Part model, mm, in its own coordinate system. Face numbers are marked on the shaded views. A direction names the side the tool comes from. Round coordinates to 2 decimals unless told otherwise and drop trailing zeros. Loops run counter-clockwise (first coordinate to the right, second up) from the corner with the lowest first, then second, coordinate; pieces in that order, holes last. Notation, with made-up numbers: (-21.75, 80) - (-2.75, 80) arc R18 ccw to (-2.75, 101) - close; hole circle Ø1 at (-33.75, 80.5). An arc over 180 degrees is marked (long way). Put each result on its own line as item: value.
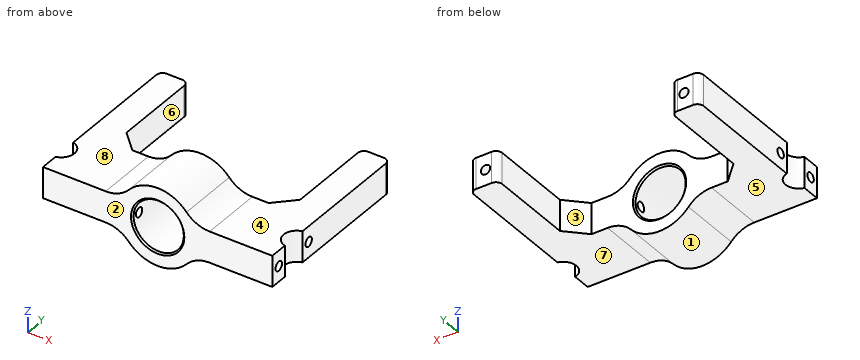
from build123d import *

# Parameters (mm, degrees)
SKETCH1_W                = 88
SKETCH1_H                = 10
BOSS_EXTRUDE1_DEPTH      = 20
SKETCH2_R                = 4.25
CUT_EXTRUDE1_DEPTH       = 11
SKETCH7_R                = 12.5
BOSS_EXTRUDE2_DEPTH      = 20
SKETCH4_R                = 8.1
CUT_EXTRUDE3_DEPTH       = 21
FILLET2_R                = 10
SKETCH9_W                = 7
SKETCH9_H                = 20
CUT_EXTRUDE6_DEPTH       = 18.5
SKETCH10_W               = 9
SKETCH10_H               = 10
BOSS_EXTRUDE3_DEPTH      = 35
SKETCH11_R               = 1.5
CUT_EXTRUDE7_DEPTH       = 20
CHAMFER1_SIZE            = 6
FILLET3_R                = 2
CHAMFER1_OF_MIRROR1_SIZE = 6
FILLET3_OF_MIRROR1_R     = 2
CHAMFER2_SIZE            = 0.5
SKETCH12_R               = 1.5
CUT_EXTRUDE8_DEPTH       = 75


with BuildPart() as part:
    # Sketch1 → Boss-Extrude1 (new body)
    with BuildSketch(Plane(origin=(0, 0, 0), x_dir=(1, 0, 0), z_dir=(0, 1, 0))):
        Rectangle(SKETCH1_W, SKETCH1_H)
    extrude(amount=BOSS_EXTRUDE1_DEPTH)

    # Sketch2 → Cut-Extrude1 (cut, through all)
    with BuildSketch(Plane.XY.offset(5)):
        with Locations((-38, 10)):
            Circle(SKETCH2_R)
        with Locations((38, 10)):
            Circle(SKETCH2_R)
    extrude(amount=-CUT_EXTRUDE1_DEPTH, mode=Mode.SUBTRACT)

    # Sketch7 → Boss-Extrude2 (add)
    with BuildSketch(Plane(origin=(0, 20, 0), x_dir=(1, 0, 0), z_dir=(0, 1, 0))):
        Circle(SKETCH7_R)
    extrude(amount=-BOSS_EXTRUDE2_DEPTH)

    # Sketch4 → Cut-Extrude3 (cut, through all)
    with BuildSketch(Plane(origin=(0, 20, 0), x_dir=(1, 0, 0), z_dir=(0, 1, 0))):
        Circle(SKETCH4_R)
    extrude(amount=-CUT_EXTRUDE3_DEPTH, mode=Mode.SUBTRACT)

    # Fillet2
    fillet2_edges = [part.edges().sort_by_distance(p)[0] for p in [
        (11.456439237, 10, -5),
        (11.456439237, 10, 5),
        (-11.456439237, 10, -5),
        (-11.456439237, 10, 5),
    ]]
    fillet(fillet2_edges, radius=FILLET2_R)

    # Sketch9 → Cut-Extrude6 (cut, through all)
    with BuildSketch(Plane.XY.offset(5)):
        with Locations((-40.5, 10)):
            Rectangle(SKETCH9_W, SKETCH9_H)
        with Locations((40.5, 10)):
            Rectangle(SKETCH9_W, SKETCH9_H)
    extrude(amount=-CUT_EXTRUDE6_DEPTH, mode=Mode.SUBTRACT)

    # Sketch10 → Boss-Extrude3 (add)
    with BuildSketch(Plane(origin=(0, 20, 0), x_dir=(1, 0, 0), z_dir=(0, 1, 0))):
        with Locations((-32.5, 0)):
            Rectangle(SKETCH10_W, SKETCH10_H)
    boss_extrude3 = extrude(amount=BOSS_EXTRUDE3_DEPTH)

    # Sketch11 → Cut-Extrude7 (cut)
    with BuildSketch(Plane(origin=(0, 55, 0), x_dir=(1, 0, 0), z_dir=(0, 1, 0))):
        with Locations((-32, 0)):
            Circle(SKETCH11_R)
    cut_extrude7 = extrude(amount=-CUT_EXTRUDE7_DEPTH, mode=Mode.SUBTRACT)

    # Chamfer1
    chamfer1_edges = [part.edges().sort_by_distance(p)[0] for p in [
        (-28, 20, 0),
    ]]
    chamfer(chamfer1_edges, length=CHAMFER1_SIZE)

    # Fillet3
    fillet3_edges = [part.edges().sort_by_distance(p)[0] for p in [
        (-37, 55, 0),
        (-28, 55, 0),
    ]]
    fillet(fillet3_edges, radius=FILLET3_R)

    # Mirror1: Boss-Extrude3, Cut-Extrude7 across plane
    add(boss_extrude3.mirror(Plane(origin=(0, 0, 0), x_dir=(0, 0, 1), z_dir=(1, 0, 0))))
    add(cut_extrude7.mirror(Plane(origin=(0, 0, 0), x_dir=(0, 0, 1), z_dir=(1, 0, 0))), mode=Mode.SUBTRACT)

    # Chamfer1 of Mirror1
    chamfer1_of_mirror1_edges = [part.edges().sort_by_distance(p)[0] for p in [
        (28, 20, 0),
    ]]
    chamfer(chamfer1_of_mirror1_edges, length=CHAMFER1_OF_MIRROR1_SIZE)

    # Fillet3 of Mirror1
    fillet3_of_mirror1_edges = [part.edges().sort_by_distance(p)[0] for p in [
        (37, 55, 0),
        (28, 55, 0),
    ]]
    fillet(fillet3_of_mirror1_edges, radius=FILLET3_OF_MIRROR1_R)

    # Chamfer2
    chamfer2_edges = [part.edges().sort_by_distance(p)[0] for p in [
        (-8.1, 0, 0),
        (-8.1, 20, 0),
    ]]
    chamfer(chamfer2_edges, length=CHAMFER2_SIZE)

    # Sketch12 → Cut-Extrude8 (cut, through all)
    with BuildSketch(Plane.ZY.offset(37)):
        with Locations((0, 3)):
            Circle(SKETCH12_R)
        with Locations((0, 17)):
            Circle(SKETCH12_R)
    extrude(amount=-CUT_EXTRUDE8_DEPTH, mode=Mode.SUBTRACT)


solid = part.part
1. Band-saw the part on B-B (y = 29.5). List the corners of the cut face in (x, z), plus the area to 3 significant figures.
A:
outline: (-37, -5) - (-28, -5) - (-28, 5) - (-37, 5) - close; (28, -5) - (37, -5) - (37, 5) - (28, 5) - close
area: 180 mm²
2. Band-saw the part on C-C (x = -32). List the corners of the cut face in (y, z), plus the area to 3 significant figures.
A:
outline: (0, -5) - (55, -5) - (55, -1.5) - (35, -1.5) - (35, 1.5) - (55, 1.5) - (55, 5) - (0, 5) - close; hole circle Ø3 at (3, 0); hole circle Ø3 at (17, 0)
area: 476 mm²
3. Band-saw the part on A-A (x = 0). List the corners of the cut face in (y, z), plus the area to 4 significant figures.
A:
outline: (0, -12.5) - (20, -12.5) - (20, -8.6) - (19.5, -8.1) - (0.5, -8.1) - (0, -8.6) - close; (0, 8.6) - (0.5, 8.1) - (19.5, 8.1) - (20, 8.6) - (20, 12.5) - (0, 12.5) - close
area: 175.5 mm²
4. Two-plate mould, pull along X, no slides. Class the marked faces 1, 2 and 3: pulls with the +X half, pulls with the -X half, needs draft (parallel to the pull), parting line crosses it, or undercut.
A:
face 1: parting line crosses it
face 2: needs draft
face 3: undercut
5. Pin check, flat tips, straight feed: P1, Ø2.5, axis at x = 32, z = 0, coming from the -Y side; P2, Ø10, axis at x = 21.5, y = 39.5, coming from the -Z side; P3, Ø5, axis at x = -29, y = 31, coming from the -Z side; P4, Ø0.9, axis at x = 32.5, z = -0.5, coming from the +Y side. Stop position of each tip, or through.
A:
P1: stops at y = 0
P2: passes through
P3: stops at z = -5
P4: stops at y = 35
6. Probe line 1 along Y through (x, z) = (14, 0); line 2 along X through (y, z) = (44.5, 0); line 3 along Z through (x, y) = (0, 6.5). List the from-to ranges inside material, lowest first. Write a range as [from, to].
A:
line 1: y = [0, 1.5], [4.5, 15.5], [18.5, 20]
line 2: x = [-37, -33.5], [-30.5, -28], [28, 30.5], [33.5, 37]
line 3: z = [-12.5, -8.1], [8.1, 12.5]
7. Band-saw the part on D-D (y = 17). List the corners of the cut face in (x, z), plus the area to 3 significant figures.
A:
outline: (-37, -5) - (-16.77, -5) arc R10 cw to (-9.32, -8.33) arc R12.5 ccw to (9.32, -8.33) arc R10 cw to (16.77, -5) - (37, -5) - (37, -1.5) - (7.96, -1.5) arc R8.1 cw to (-7.96, -1.5) - (-37, -1.5) - close; (-37, 1.5) - (-7.96, 1.5) arc R8.1 cw to (7.96, 1.5) - (37, 1.5) - (37, 5) - (16.77, 5) arc R10 cw to (9.32, 8.33) arc R12.5 ccw to (-9.32, 8.33) arc R10 cw to (-16.77, 5) - (-37, 5) - close
area: 623 mm²
8. Tool access for the marked faces 4, 5, 6, 7 and 8: list every direction of +Z, -Z, +X, -X, +Y, -Y with a clear straight run to the whole face (end or side of a thin tool).
A:
face 4: +Z, +X, +Y, -Y
face 5: -Z, -X, +Y, -Y
face 6: +Z, -Z, +Y
face 7: -Z, +X, +Y, -Y
face 8: +Z, -X, +Y, -Y
